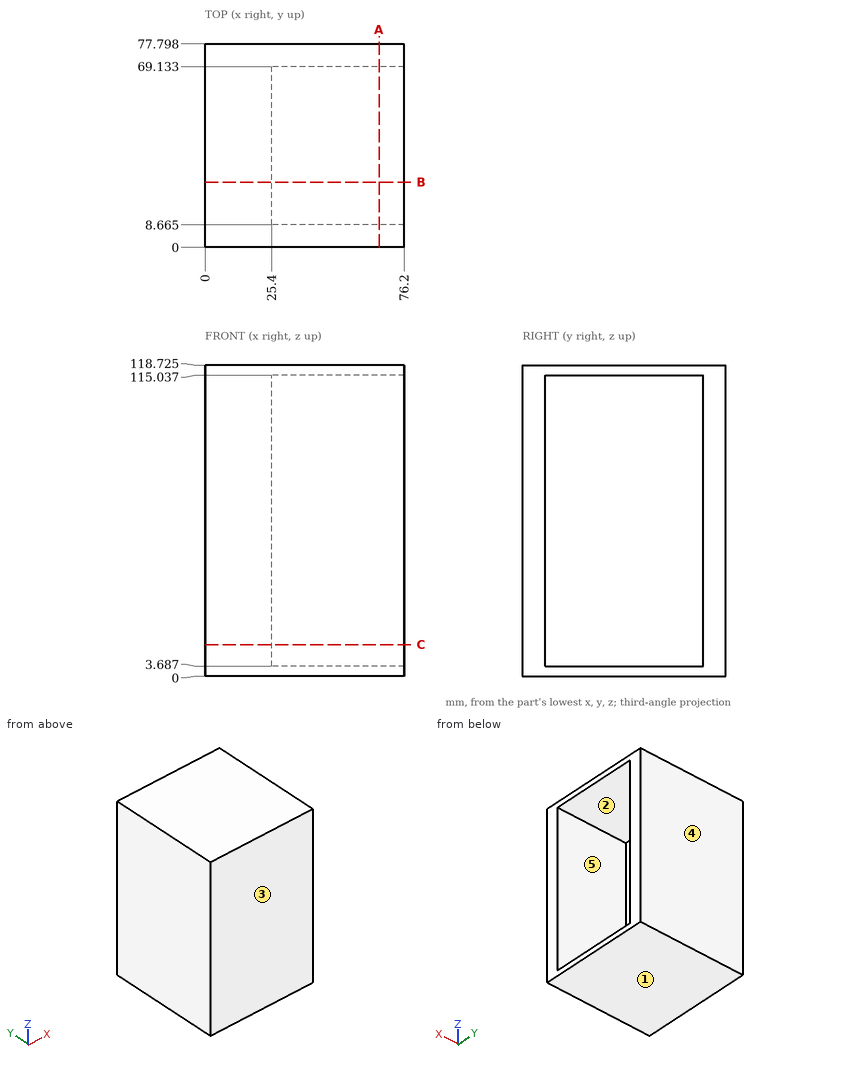
For this review, use the dimensioned drawing (mm, ordinates from the lowest corner) and the shaded views. A direction names the side the tool comes from. Round coordinates to 2 decimals unless told otherwise and drop trailing zeros. Order: outer loops, then holes, each group sorted by start corner. A loop starts at its lowest first (then second) coordinate and runs counter-clockwise, first axis right, second up. Notation, with made-up numbers: (66.5, 11) -> (105.5, 11) arc R27 ccw to (105.5, 35) -> close; hole circle Ø11 at (28.5, -33.5). An arc over 180 degrees is marked (long way). Use CSV: the item, a comma, the result in double quotes. Start each with the question number.
(1) Insertion check: pin 1 (10 mm diameter, centred on y = 62.5, z = 86.5, fed in from +X). The pin has a flat end and moves straight along its axis. Give the tip position at first contact, or say it passes through.
(2) Mouldability with a two-part tool opening along Y and no side actions: class the marked faces 1, 2 and 3 as pulls with the +Y half, pulls with the -Y half, needs draft (parallel to the pull), parting line crosses it, or undercut.
(3) Wall thickness on probe 1 along Y at (x, z) = (33, 77) (1 decimal); probe 2 along Z at (x, y) = (30, 63) (1 decimal); probe 3 along X at (y, z) = (49.5, 18): over which ranges is each line inside the solid? List them lowest first. Write a range as from..to.
(4) Tool access review of the marked faces 4 and 5: name each direction out of +Z, -Z, +X, -X, +Y, -Y from which nothing blocks a thin tool from reaching the whole face with its end or side.
(5) Consider section B-B on y = 25. Write out the cut boundary in (x, z) (1 decimal), and give its area (3 significant figures).
(6) Consider section A-A on x = 66.5. Write out the cut boundary in (y, z) (1 decimal), and give its area (3 significant figures).
(7) Consider section C-C on z = 12. Write out the cut boundary in (x, y) (1 decimal).
Responses:
1,pin 1,"x = 25.4"
2,face 1,"needs draft"
2,face 2,"undercut"
2,face 3,"pulls with the -Y half"
3,probe 1,"0..8.7, 69.1..77.8"
3,probe 2,"0..3.7, 115..118.7"
3,probe 3,"0..25.4"
4,face 4,"+Z, -Z, +X, -X, +Y"
4,face 5,"+X"
5,outline,"(0, 0) -> (76.2, 0) -> (76.2, 3.7) -> (25.4, 3.7) -> (25.4, 115) -> (76.2, 115) -> (76.2, 118.7) -> (0, 118.7) -> close"
5,area,"3,390 mm²"
6,outline,"(0, 0) -> (77.8, 0) -> (77.8, 118.7) -> (0, 118.7) -> close; hole (8.7, 3.7) -> (69.1, 3.7) -> (69.1, 115) -> (8.7, 115) -> close"
6,area,"2,500 mm²"
7,outline,"(0, 0) -> (76.2, 0) -> (76.2, 8.7) -> (25.4, 8.7) -> (25.4, 69.1) -> (76.2, 69.1) -> (76.2, 77.8) -> (0, 77.8) -> close"
